Answer from the drawing. Dimensions are ordinates in mm from the lowest x, y and z of the part. Coordinates: 2 decimals unless noted, no trailing zeros. Write each loop counter-clockwise with the first axis right and the second up, starting at its lowest first coordinate (ties: lowest second). Pieces come first, ordered by that corner, then holes.
(1) Determine the mould class of the marked faces 1, 2 and 3 for opening direction Z: pulls with the +Z half, pulls with the -Z half, needs draft (parallel to the pull), parting line crosses it, or undercut.
(2) Straight lines are drawn through the part: line 1 along Z through (x, y) = (8.5, 4.6); line 2 along X through (y, z) = (0.5, 12.25); line 3 along Y through (x, z) = (9.75, 5). For each, find the intervals that lie inside material, in ascending order.
(3) Given pin 1 (2 mm diameter, centred on y = 2.5, z = 11.5, fed in from -X); pin 2 (1 mm diameter, centred on x = 13, z = 9.5, fed in from -Y); pin 3 (8 mm diameter, centred on x = 11.5, z = 7.5, fed in from +Y); pin 4 (9 mm diameter, centred on x = 8.5, z = 8.5, fed in from -Y), each flat-ended and moving along its own axis, determine where each tip first touches the part or whether it passes through.
(4) The part is cut by section C-C, the plane y = 7.25. Determine the outline of the cut face in (x, z), and give its area (3 significant figures).
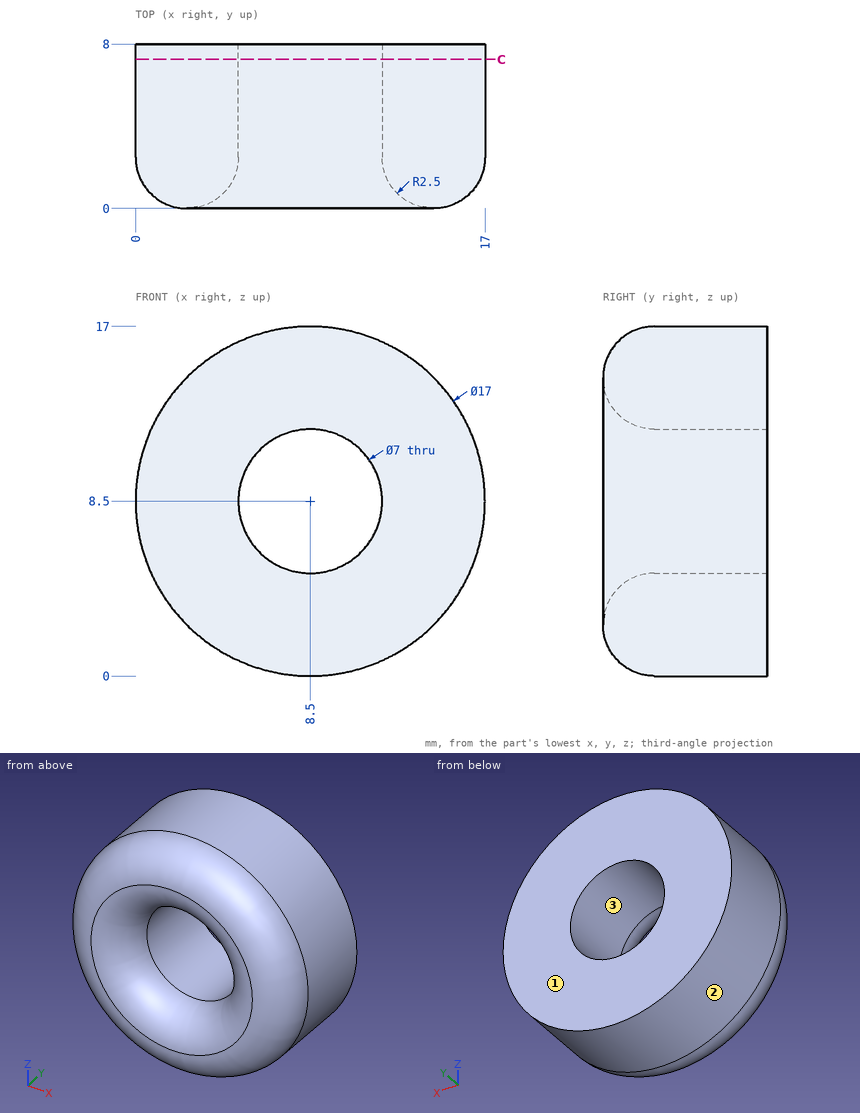
Computed:
1. face 1: needs draft
1. face 2: parting line crosses it
1. face 3: undercut
2. line 1: z = 0 to 5, 12 to 17
2. line 2: x = 2 to 6.01, 10.99 to 15
2. line 3: y = 1.48 to 8
3. pin 1: stops at x = 0.24
3. pin 2: stops at y = 0.16
3. pin 3: stops at y = 8
3. pin 4: stops at y = 0.5
4. outline: circle Ø17 at (8.5, 8.5); hole circle Ø7 at (8.5, 8.5)
4. area: 188 mm2
